from build123d import *

# Parameters (mm, degrees)
EXTRUDE_1_DEPTH     = 57.7
EXTRUDE_2_DEPTH     = 30.8
SKETCH_5_R          = 4
CUT_EXTRUDE_1_DEPTH = 15
FILLET_1_R          = 10
SKETCH_6_W          = 6
SKETCH_6_H          = 1.5
EXTRUDE_3_DEPTH     = 6
EXTRUDE_START       = -37
SKETCH_6_3_W        = 6
SKETCH_6_3_H        = 1.5
EXTRUDE_4_DEPTH     = 6
SKETCH_7_R          = 2
CUT_EXTRUDE_2_DEPTH = 6
SKETCH_8_W          = 14.5
SKETCH_8_H          = 25.5
CUT_EXTRUDE_3_DEPTH = 2
SKETCH_9_R          = 13
CUT_EXTRUDE_4_DEPTH = 44.487239508


with BuildPart() as part:
    # 스케치1 → 보스-돌출1 (new body)
    with BuildSketch(Plane.XY):
        with BuildLine():
            Line((-13.5, 0), (-18.5, 0))
            Line((-18.5, 0), (-18.5, -18.5))
            Line((-18.5, -18.5), (18.5, -18.5))
            Line((18.5, -18.5), (18.5, 0))
            Line((18.5, 0), (13.5, 0))
            ThreePointArc((13.5, 0), (0, -13.5), (-13.5, 0))
        make_face()
    extrude(amount=-EXTRUDE_1_DEPTH)

    # 스케치3 → 보스-돌출2 (add)
    with BuildSketch(Plane.XY.offset(-26.9)):
        with BuildLine():
            Line((-13.5, 0), (-11.5, 0))
            ThreePointArc((-11.5, 0), (0, -11.5), (11.5, 0))
            Line((11.5, 0), (13.5, 0))
            ThreePointArc((13.5, 0), (0, -13.5), (-13.5, 0))
        make_face()
    extrude(amount=-EXTRUDE_2_DEPTH)

    # 스케치5 → 컷-돌출1 (cut)
    with BuildSketch(Plane.ZY.offset(18.5)):
        with Locations((-21.9, 0)):
            Circle(SKETCH_5_R)
    extrude(amount=-CUT_EXTRUDE_1_DEPTH, mode=Mode.SUBTRACT)

    # 필렛1
    fillet_1_edges = [part.edges().sort_by_distance(p)[0] for p in [
        (18.5, -18.5, -28.85),
        (-18.5, -18.5, -28.85),
    ]]
    fillet(fillet_1_edges, radius=FILLET_1_R)

    # 스케치6 → 보스-돌출3 (add)
    with BuildSketch(Plane(origin=(18.5, 0, 0), x_dir=(0, 0, -1), z_dir=(1, 0, 0))):
        with Locations((37.7, -0.75)):
            Rectangle(SKETCH_6_W, SKETCH_6_H)
        with Locations((9, -0.75)):
            Rectangle(SKETCH_6_W, SKETCH_6_H)
    extrude(amount=EXTRUDE_3_DEPTH)

    # 스케치6<3> → 보스-돌출4 (add)
    with BuildSketch(Plane(origin=(18.5, 0, 0), x_dir=(0, 0, -1), z_dir=(1, 0, 0)).offset(EXTRUDE_START)):
        with Locations((37.7, -0.75)):
            Rectangle(SKETCH_6_3_W, SKETCH_6_3_H)
        with Locations((9, -0.75)):
            Rectangle(SKETCH_6_3_W, SKETCH_6_3_H)
    extrude(amount=-EXTRUDE_4_DEPTH)

    # 스케치7 → 컷-돌출2 (cut)
    with BuildSketch(Plane(origin=(0, 0, 0), x_dir=(1, 0, 0), z_dir=(0, 1, 0))):
        with Locations(Location((21.5, 9, 0), (0, 0, 270))):
            Circle(SKETCH_7_R)
        with Locations(Location((21.5, 37.7, 0), (0, 0, 270))):
            Circle(SKETCH_7_R)
        with Locations(Location((-21.5, 9, 0), (0, 0, 180))):
            Circle(SKETCH_7_R)
        with Locations((-21.5, 37.7)):
            Circle(SKETCH_7_R)
    extrude(amount=-CUT_EXTRUDE_2_DEPTH, mode=Mode.SUBTRACT)

    # 스케치8 → 컷-돌출3 (cut)
    with BuildSketch(Plane.XZ.offset(18.5)):
        with Locations((0, -42.95)):
            Rectangle(SKETCH_8_W, SKETCH_8_H)
    extrude(amount=-CUT_EXTRUDE_3_DEPTH, mode=Mode.SUBTRACT)

    # 스케치9 → 컷-돌출4 (cut, through all)
    with BuildSketch(Plane.XY.offset(-26.9)):
        Circle(SKETCH_9_R)
    extrude(amount=-CUT_EXTRUDE_4_DEPTH, mode=Mode.SUBTRACT)


solid = part.part
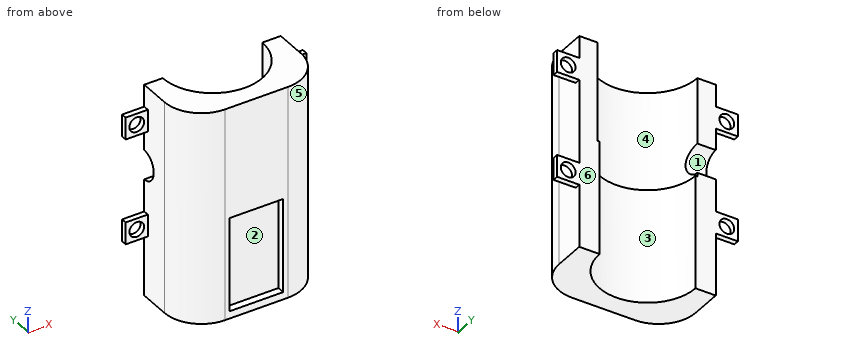
Read the model definition and answer for the solid it produces. Units are mm, in the model's axes. Face numbers are marked on the shaded views. A direction names the side the tool comes from. Give positions to 0.01 mm unless a question says otherwise; leave off trailing zeros. Loops run counter-clockwise (first coordinate to the right, second up) from the corner with the lowest first, then second, coordinate; pieces in that order, holes last. Notation, with made-up numbers: (42.5, 81) -> (57.5, 81) arc R17 cw to (57.5, 97) -> close; hole circle Ø6 at (31, -16.75). An arc over 180 degrees is marked (long way). Use a Markdown table: item, result.
Q1. Determine the mould class of the marked faces 4, 5 and 6 for opening direction X: pulls with the +X half, pulls with the -X half, needs draft (parallel to the pull), parting line crosses it, or undercut.
Solved:
| item | result |
|---|---|
| face 4 | undercut |
| face 5 | pulls with the +X half |
| face 6 | needs draft |
Q2. A tool of negligible diameter and unlimited length cuts with its end or side. For the marked faces 1, 2 and 3, from which of +Z, -Z, +X, -X, +Y, -Y can it reach the whole face along a straight path? Write none if from no direction.
Solved:
| item | result |
|---|---|
| face 1 | -X, +Y |
| face 2 | -Y |
| face 3 | +Z, -Z, +Y |
Q3. Each of these flat-tipped pins is pushed along its axis until it touches: pin 1 (4.5 mm diameter, centred on x = 21.5, z = -37.7, fed in from +Y); pin 2 (0.6 mm diameter, centred on y = -17.5, z = -42.5, fed in from +X); pin 3 (6 mm diameter, centred on y = -9, z = -17.5, fed in from +X); pin 4 (1.2 mm diameter, centred on x = 21.5, y = -1, fed in from +Z). Where does it stop, or does it pass through?
Solved:
| item | result |
|---|---|
| pin 1 | stops at y = 0 |
| pin 2 | stops at x = 13.43 |
| pin 3 | stops at x = 18.5 |
| pin 4 | stops at z = -6 |
Q4. Section C-C, the plane z = -21.9 is taken. Determine the outline of the cut face in (x, y), then the cut area to 3 significant figures.
Solved:
| item | result |
|---|---|
| outline | (-18.5, -8.5) arc R10 ccw to (-8.5, -18.5) -> (8.5, -18.5) arc R10 ccw to (18.5, -8.5) -> (18.5, 0) -> (13.5, 0) arc R13.5 cw to (-12.89, -4) -> (-18.5, -4) -> close |
| area | 335 mm^2 |
Q5. Section D-D, the plane x = 0 is taken. Determine the outline of the cut face in (y, z), then the cut area to 3 significant figures.
Solved:
| item | result |
|---|---|
| outline | (-18.5, -57.7) -> (-13, -57.7) -> (-13, -26.9) -> (-13.5, -26.9) -> (-13.5, 0) -> (-18.5, 0) -> (-18.5, -30.2) -> (-16.5, -30.2) -> (-16.5, -55.7) -> (-18.5, -55.7) -> close |
| area | 253 mm^2 |
Q6. Section B-B, the plane y = -4.75 is taken. Determine the outline of the cut face in (x, z).
Solved:
| item | result |
|---|---|
| outline | (-18.5, -57.7) -> (-12.1, -57.7) -> (-12.1, -26.9) -> (-12.64, -26.9) -> (-12.64, 0) -> (-18.5, 0) -> close; (12.1, -57.7) -> (18.5, -57.7) -> (18.5, 0) -> (12.64, 0) -> (12.64, -26.9) -> (12.1, -26.9) -> close |
Q7. Section A-A, the plane x = 21.5 is taken. Determine the outline of the cut face in (y, z), then the cut area to 3 significant figures.
Solved:
| item | result |
|---|---|
| outline | (-1.5, -40.7) -> (0, -40.7) -> (0, -39.7) -> (-1.5, -39.7) -> close; (-1.5, -35.7) -> (0, -35.7) -> (0, -34.7) -> (-1.5, -34.7) -> close; (-1.5, -12) -> (0, -12) -> (0, -11) -> (-1.5, -11) -> close; (-1.5, -7) -> (0, -7) -> (0, -6) -> (-1.5, -6) -> close |
| area | 6.00 mm^2 |
Q8. Find the intervals of material crossed by line 1 along Z through (x, y) = (-21.5, -1.05); line 2 along X through (y, z) = (-1.2, -37.7); line 3 along X through (y, z) = (-0.75, -37.7), in increasing order.
Solved:
| item | result |
|---|---|
| line 1 | z = -40.7 to -39.7, -35.7 to -34.7, -12 to -11, -7 to -6 |
| line 2 | x = -24.5 to -23.5, -19.5 to -12.94, 12.94 to 19.5, 23.5 to 24.5 |
| line 3 | x = -24.5 to -23.5, -19.5 to -12.98, 12.98 to 19.5, 23.5 to 24.5 |
